Geometry check sheet. Reference: drawing and pictorial views, mm from the part's lowest x, y, z. A direction names the side the tool comes from. Give positions to 0.01 mm unless a question says otherwise; leave off trailing zeros. Write each loop counter-clockwise with the first axis right and the second up, starting at its lowest first coordinate (ties: lowest second). Pieces come first, ordered by that corner, then holes. Notation, with made-up numbers: (11.25, 17.25) -> (32.25, 17.25) arc R16 cw to (32.25, 31.25) -> close; hole circle Ø1 at (-26, 26). An arc over 180 degrees is marked (long way). Use a Markdown table: item, result. Add a question column.
1. Cross-section at B-B (x = 6.5). Enter the section's corners in (y, z).
2. Cross-section at D-D (z = 10). Enter the section's corners in (x, y), then the cut area to 3 significant figures.
3. Set-up check for the marked faces 1, 2 and 3: record each of +Z, -Z, +X, -X, +Y, -Y from which the full face is reachable in a straight line by a thin tool's end or side.
4. Cross-section at C-C (y = 11.5). Enter the section's corners in (x, z), then the cut area to 3 significant figures.
5. Gauge pin test, flat ends, axial feed: P1, Ø4, axis at x = 42, z = 11, coming from the -Y side; P2, Ø3, axis at y = 18, z = 8, coming from the -X side; P3, Ø12, axis at x = 38.5, z = 16.5, coming from the -Y side. Record the tip position at first contact, or that the pin passes through.
6. Cross-section at A-A (z = 18.75). Enter the section's corners in (x, y).
7. Release check for a two-part mould opening along Z. For the marked faces 4, 5, 6 and 7 record: released by +Z, released by -Z, zero draft, split by the parting line, or undercut.
8. Scan lines: probe 1 along X at (y, z) = (20.5, 7.5); probe 2 along Z at (x, y) = (2, 17); probe 3 along Y at (x, z) = (6.5, 1.4). Record each from-to range of solid material in increasing order. Write a range as [from, to].
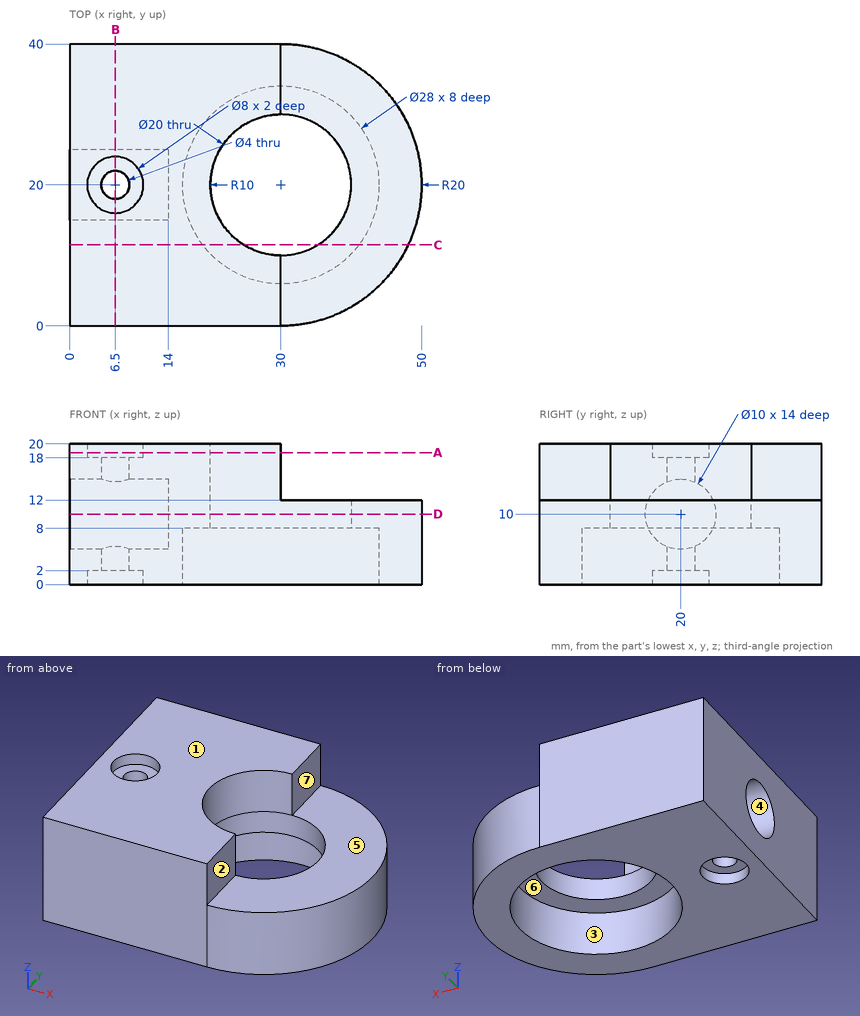
Worked answers:
| question | item | result |
|---|---|---|
| 1 | outline | (0, 0) -> (16, 0) -> (16, 2) -> (18, 2) -> (18, 5.42) arc R5 cw to (18, 14.58) -> (18, 18) -> (16, 18) -> (16, 20) -> (0, 20) -> close; (22, 2) -> (24, 2) -> (24, 0) -> (40, 0) -> (40, 20) -> (24, 20) -> (24, 18) -> (22, 18) -> (22, 14.58) arc R5 cw to (22, 5.42) -> close |
| 2 | outline | (0, 0) -> (30, 0) arc R20 ccw to (30, 40) -> (0, 40) -> (0, 25) -> (14, 25) -> (14, 15) -> (0, 15) -> close; hole circle Ø20 at (30, 20) |
| 2 | area | 1,370 mm² |
| 3 | face 1 | +Z, +X, -X, +Y, -Y |
| 3 | face 2 | +Z, +X, +Y, -Y |
| 3 | face 3 | -Z |
| 4 | outline | (0, 0) -> (18.88, 0) -> (18.88, 8) -> (24.73, 8) -> (24.73, 20) -> (0, 20) -> close; (35.27, 8) -> (41.12, 8) -> (41.12, 0) -> (48.1, 0) -> (48.1, 12) -> (35.27, 12) -> close |
| 4 | area | 555 mm² |
| 5 | P1 | stops at y = 2.68 |
| 5 | P2 | stops at x = 14 |
| 5 | P3 | stops at y = 0.52 |
| 6 | outline | (0, 0) -> (30, 0) -> (30, 10) arc R10 cw to (30, 30) -> (30, 40) -> (0, 40) -> close; hole circle Ø8 at (6.5, 20) |
| 7 | face 4 | undercut |
| 7 | face 5 | released by +Z |
| 7 | face 6 | released by -Z |
| 7 | face 7 | zero draft |
| 8 | probe 1 | x = [14, 16.01], [43.99, 49.99] |
| 8 | probe 2 | z = [0, 6], [14, 20] |
| 8 | probe 3 | y = [0, 16], [24, 40] |
